For this review, take the finished solid that the model builds, in its own axes (mm). Face numbers are marked on the shaded views. A direction names the side the tool comes from. Coordinates: 2 decimals unless noted, no trailing zeros. Order: outer loops, then holes, each group sorted by start corner. A loop starts at its lowest first (then second) coordinate and runs counter-clockwise, first axis right, second up.
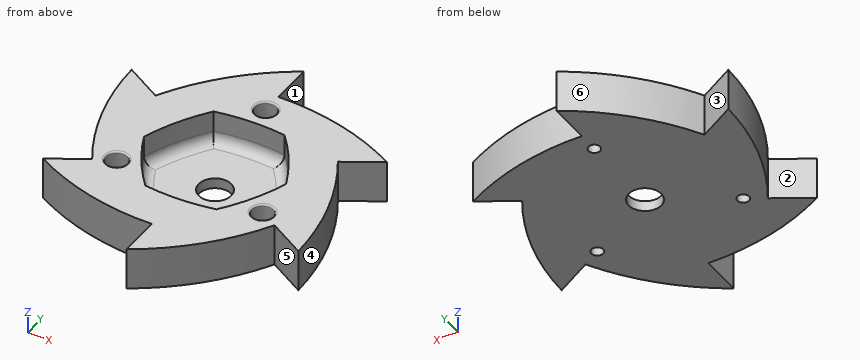
from build123d import *

# Parameters (mm, degrees)
BOSS_EXTRUDE1_DEPTH             = 6.35
BOSS_EXTRUDE1_DEPTH_BACK        = 6.35
BOSS_EXTRUDE2_START             = -12.7
BOSS_EXTRUDE2_DEPTH             = 12.7
CUT_EXTRUDE1_DEPTH              = 9.525
FILLET1_R                       = 3.175
W_0_386_DIAMETER_HOLE1_D        = 9.8044
F_9_64_0_14063_DIAMETER_HOLE1_D = 3.572002
CIRPATTERN1_COUNT               = 3
F_0_257_DIAMETER_HOLE1_D        = 6.5278
F_0_257_DIAMETER_HOLE1_DEPTH    = 9.652
FILLET2_R                       = 0.5


with BuildPart() as part:
    # Sketch1 → Boss-Extrude1 (new, two sides: drawn at the far end of the back side and taken through both)
    with BuildSketch(Plane.XY.offset(-BOSS_EXTRUDE1_DEPTH_BACK)):
        with BuildLine():
            Line((27.49630657, 15.875), (38.494829198, 22.225))
            ThreePointArc((38.494829198, 22.225), (19.878280804, 29.537115412), (0, 31.75))
            Line((0, 31.75), (0, 44.45))
            ThreePointArc((0, 44.45), (-15.640751899, 31.983653865), (-27.49630657, 15.875))
            Line((-27.49630657, 15.875), (-38.494829198, 22.225))
            ThreePointArc((-38.494829198, 22.225), (-35.519032703, 2.446538454), (-27.49630657, -15.875))
            Line((-27.49630657, -15.875), (-38.494829198, -22.225))
            ThreePointArc((-38.494829198, -22.225), (-19.878280804, -29.537115412), (0, -31.75))
            Line((0, -31.75), (0, -44.45))
            ThreePointArc((0, -44.45), (15.640751899, -31.983653865), (27.49630657, -15.875))
            Line((27.49630657, -15.875), (38.494829198, -22.225))
            ThreePointArc((38.494829198, -22.225), (35.519032703, -2.446538454), (27.49630657, 15.875))
        make_face()
        with BuildLine():
            ThreePointArc((-11.129967969, 17.779280801), (-16.817028225, 8.924127912), (-20.962292819, -0.749194604))
            ThreePointArc((-20.962292819, -0.749194604), (-16.137035591, -10.101909703), (-9.83232485, -18.528475405))
            ThreePointArc((-9.83232485, -18.528475405), (0.679992634, -19.026037615), (11.129967969, -17.779280801))
            ThreePointArc((11.129967969, -17.779280801), (16.817028225, -8.924127912), (20.962292819, 0.749194604))
            ThreePointArc((20.962292819, 0.749194604), (16.137035591, 10.101909703), (9.83232485, 18.528475405))
            ThreePointArc((9.83232485, 18.528475405), (-0.679992634, 19.026037615), (-11.129967969, 17.779280801))
        make_face(mode=Mode.SUBTRACT)
    extrude(amount=BOSS_EXTRUDE1_DEPTH + BOSS_EXTRUDE1_DEPTH_BACK)

    # Sketch3 → Boss-Extrude2 (add)
    with BuildSketch(Plane.XY.offset(6.35).offset(BOSS_EXTRUDE2_START)):
        with BuildLine():
            ThreePointArc((-11.129967969, 17.779280801), (-16.817028225, 8.924127912), (-20.962292819, -0.749194604))
            ThreePointArc((-20.962292819, -0.749194604), (-16.137035591, -10.101909703), (-9.83232485, -18.528475405))
            ThreePointArc((-9.83232485, -18.528475405), (0.679992634, -19.026037615), (11.129967969, -17.779280801))
            ThreePointArc((11.129967969, -17.779280801), (16.817028225, -8.924127912), (20.962292819, 0.749194604))
            ThreePointArc((20.962292819, 0.749194604), (16.137035591, 10.101909703), (9.83232485, 18.528475405))
            ThreePointArc((9.83232485, 18.528475405), (-0.679992634, 19.026037615), (-11.129967969, 17.779280801))
        make_face()
    extrude(amount=BOSS_EXTRUDE2_DEPTH)

    # Sketch3_2 → Cut-Extrude1 (cut)
    with BuildSketch(Plane.XY.offset(6.35)):
        with BuildLine():
            ThreePointArc((-11.129967969, 17.779280801), (-16.817028225, 8.924127912), (-20.962292819, -0.749194604))
            ThreePointArc((-20.962292819, -0.749194604), (-16.137035591, -10.101909703), (-9.83232485, -18.528475405))
            ThreePointArc((-9.83232485, -18.528475405), (0.679992634, -19.026037615), (11.129967969, -17.779280801))
            ThreePointArc((11.129967969, -17.779280801), (16.817028225, -8.924127912), (20.962292819, 0.749194604))
            ThreePointArc((20.962292819, 0.749194604), (16.137035591, 10.101909703), (9.83232485, 18.528475405))
            ThreePointArc((9.83232485, 18.528475405), (-0.679992634, 19.026037615), (-11.129967969, 17.779280801))
        make_face()
    extrude(amount=-CUT_EXTRUDE1_DEPTH, mode=Mode.SUBTRACT)

    # Fillet1
    fillet1_edges = [part.edges().sort_by_distance(p)[0] for p in [
        (-0.679992634, 19.026037615, -3.175),
        (16.137035591, 10.101909703, -3.175),
        (16.817028225, -8.924127912, -3.175),
        (0.679992634, -19.026037615, -3.175),
        (-16.137035591, -10.101909703, -3.175),
        (-16.817028225, 8.924127912, -3.175),
    ]]
    fillet(fillet1_edges, radius=FILLET1_R)

    # W _0.386_ Diameter Hole1 (through all)
    with Locations(Plane.XY.offset(-3.175)):
        with Locations((0, 0)):
            Hole(W_0_386_DIAMETER_HOLE1_D / 2)

    # 9_64 _0.14063_ Diameter Hole1 (through all)
    with Locations(Plane(origin=(0, 0, -6.35), x_dir=(-1, 0, 0), z_dir=(0, 0, -1))):
        with Locations((0, 25.4)):
            f_9_64_0_14063_diameter_hole1 = Hole(F_9_64_0_14063_DIAMETER_HOLE1_D / 2)

    # CirPattern1: 9_64 _0.14063_ Diameter Hole1 ×3 about axis
    cirpattern1_axis = Axis((0, 0, 0), (0, 0, 1))
    for i in range(1, CIRPATTERN1_COUNT):
        add(f_9_64_0_14063_diameter_hole1.rotate(cirpattern1_axis, i * 360 / CIRPATTERN1_COUNT), mode=Mode.SUBTRACT)

    # F _0.257_ Diameter Hole1
    with Locations(Plane.XY.offset(6.35)):
        with Locations((0, 25.4), (21.997045256, -12.7), (-21.997045256, -12.7)):
            Hole(F_0_257_DIAMETER_HOLE1_D / 2, depth=F_0_257_DIAMETER_HOLE1_DEPTH)

    # Fillet2
    fillet2_edges = [part.edges().sort_by_distance(p)[0] for p in [
        (-18.733145256, -12.7, 6.35),
        (25.260945256, -12.7, 6.35),
        (3.2639, 25.4, 6.35),
    ]]
    fillet(fillet2_edges, radius=FILLET2_R)


solid = part.part
1. The part is to be moulded in two halves that separate along Y. For the marked faces 1, 2 and 3, say which applies: +Y half, -Y half, draft (parallel to the pull), parting line (faces both ways), or undercut.
Answer below:
face 1: draft
face 2: undercut
face 3: +Y half
2. Take a section at A-A, the plane z = 2. Give the boundary of the cut face in (x, y) (3 decimals).
Answer below:
outline: (-38.495, -22.225) arc R76.155 ccw to (0, -31.75) - (0, -44.45) arc R76.155 ccw to (27.496, -15.875) - (38.495, -22.225) arc R76.155 ccw to (27.496, 15.875) - (38.495, 22.225) arc R76.155 ccw to (0, 31.75) - (0, 44.45) arc R76.155 ccw to (-27.496, 15.875) - (-38.495, 22.225) arc R76.155 ccw to (-27.496, -15.875) - close; hole circle Ø6.528 at (-21.997, -12.7); hole (-20.962, -0.749) arc R63.455 ccw to (-9.832, -18.528) arc R63.455 ccw to (11.13, -17.779) arc R63.455 ccw to (20.962, 0.749) arc R63.455 ccw to (9.832, 18.528) arc R63.455 ccw to (-11.13, 17.779) arc R63.455 ccw to start; hole circle Ø6.528 at (0, 25.4); hole circle Ø6.528 at (21.997, -12.7)
3. Take a section at C-C, the plane x = 32. Give the boundary of the cut face in (y, z), plus the area to 3 significant figures.
Answer below:
outline: (-18.48, -6.35) - (7.23, -6.35) - (7.23, 6.35) - (-18.48, 6.35) - close; (18.48, -6.35) - (25.43, -6.35) - (25.43, 6.35) - (18.48, 6.35) - close
area: 415 mm2
4. Take a section at B-B, the plane y = 25.4. Give the boundary of the cut face in (x, z).
Answer below:
outline: (-21.29, -6.35) - (-1.79, -6.35) - (-1.79, -3.3) - (-3.26, -3.3) - (-3.26, 5.85) arc R0.5 ccw to (-3.76, 6.35) - (-21.29, 6.35) - close; (1.79, -6.35) - (32.07, -6.35) - (32.07, 6.35) - (3.76, 6.35) arc R0.5 ccw to (3.26, 5.85) - (3.26, -3.3) - (1.79, -3.3) - close
5. To check wall thickness, follow L1, parallel to X at y = -14.5, z = -2.5; L2, parallel to Z at x = 7, y = 11 (3 decimals); L3, parallel to Y at x = -28.5, z = -5. State the ranges of each line that lie inside material, in increasing order.
Answer below:
L1: x = -28.31 to -24.72, -19.27 to -11.59, 12.01 to 19.27, 24.72 to 37.96
L2: z = -6.35 to -3.175
L3: y = -26.85 to -16.45, -14.17 to 16.45
6. Take a section at D-D, the plane y = -12.7. Give the number of separate pieces and of enclosed holes in the cut face, plus the area to 3 significant figures.
Answer below:
separate pieces: 3
enclosed holes: 0
area: 432 mm2
7. Clearance check with flat-ended pins moving along their axes: pin 1 Ø6 at (y, z) = (-18.5, 4) entering from -X; pin 2 Ø5.5 at (x, y) = (0, 25.4) entering from +Z; pin 3 Ø3 at (y, z) = (-34.5, 0) entering from -X. State where each tip first meets the part, or that it passes through.
Answer below:
pin 1: stops at x = -37.24
pin 2: stops at z = -3.3
pin 3: stops at x = 0
8. Machinability: for the marked faces 4, 5 and 6, which of the approach directions +Z, -Z, +X, -X, +Y, -Y give a long, thin tool a straight path to every point of the face, cutting with its end or side? Answer none if there is none.
Answer below:
face 4: +Z, -Z, +X
face 5: +Z, -Z, -Y
face 6: +Z, -Z, +Y
